Part model, mm, in its own coordinate system. A direction names the side the tool comes from. Give positions to 0.01 mm unless a question says otherwise; leave off trailing zeros. Write each loop counter-clockwise with the first axis right and the second up, starting at its lowest first coordinate (ties: lowest second). Pieces come first, ordered by that corner, then holes. Notation, with made-up numbers: M 34.25,14 L 85.25,14 A26 ccw 85.25,44 Z; hole C 87.5,4.5 d11. An arc over 180 degrees is marked long. Write item = value, one per line. Start each with the question number.
Autodesk Inventor part; units mm, degrees
ref_plane "YZ Plane" through (0, 0, 0) normal (1, 0, 0) x (0, 1, 0)
ref_plane "XZ Plane" through (0, 0, 0) normal (0, 1, 0) x (-1, 0, 0)
ref_plane "XY Plane" through (0, 0, 0) normal (0, 0, 1) x (1, 0, 0)
sketch "Sketch1" plane through (0, 0, 0) normal (0, 0, 1) x (1, 0, 0)
  line L0 (-20.5, -19.5) -> (20.5, -19.5)
  line L1 (20.5, -19.5) -> (20.5, 19.5)
  line L2 (20.5, 19.5) -> (-20.5, 19.5)
  line L3 (-20.5, 19.5) -> (-20.5, -19.5)
  line L4 (-20.5, -19.5) -> (20.5, 19.5) construction
  line L5 (20.5, -19.5) -> (-20.5, 19.5) construction
  line L6 (-17, -17) -> (17, -17) construction
  line L7 (17, -17) -> (17, 17) construction
  line L8 (17, 17) -> (-17, 17) construction
  line L9 (-17, 17) -> (-17, -17) construction
  line L10 (-17, -17) -> (17, 17) construction
  line L11 (17, -17) -> (-17, 17) construction
  circle A0 centre (-17, 17) radius 1.5
  circle A1 centre (17, 17) radius 1.5
  circle A2 centre (17, -17) radius 1.5
  circle A3 centre (-17, -17) radius 1.5
  point P0 (0, 0)
  dimension "d0" = 41
  dimension "d1" = 39
  dimension "d2" = 34
  dimension "d3" = 34
  dimension "d4" = 3
extrude "Extrusion1" add sketch "Sketch1" against normal blind 10
sketch "Sketch2" plane through (0, 0, 0) normal (0, 0, 1) x (1, 0, 0)
  line L0 (-14, -14) -> (14, -14)
  line L1 (14, -14) -> (14, 14)
  line L2 (14, 14) -> (-14, 14)
  line L3 (-14, 14) -> (-14, -14)
  line L4 (-14, -14) -> (14, 14) construction
  line L5 (14, -14) -> (-14, 14) construction
  point P0 (0, 0)
  dimension "d7" = 28
  dimension "d8" = 28
extrude "Extrusion2" add sketch "Sketch2" along normal blind 7
sketch "Sketch3" plane through (0, 0, 7) normal (0, 0, 1) x (1, 0, 0)
  circle A0 centre (0, 0) radius 7.1
  dimension "d11" = 14.2
extrude "Extrusion3" add sketch "Sketch3" along normal blind 20
sketch "Sketch4" plane through (0, 0, -10) normal (0, 0, -1) x (-1, 0, 0)
  line L0 (-20.5, 19.5) -> (-20.5, -19.5)
  line L1 (-20.5, 19.5) -> (-13.5, 19.5)
  line L2 (-13.5, 19.5) -> (-13.5, 12.5)
  line L3 (-13.5, 12.5) -> (-20.5, 12.5)
  line L4 (-20.5, 12.5) -> (-20.5, 19.5)
  line L5 (20.5, 19.5) -> (-20.5, 19.5)
  line L6 (20.5, 19.5) -> (13.5, 19.5)
  line L7 (13.5, 19.5) -> (13.5, 12.5)
  line L8 (13.5, 12.5) -> (20.5, 12.5)
  line L9 (20.5, 12.5) -> (20.5, 19.5)
  line L10 (20.5, 19.5) -> (20.5, -19.5)
  line L11 (20.5, -19.5) -> (13.5, -19.5)
  line L12 (13.5, -19.5) -> (13.5, -12.5)
  line L13 (13.5, -12.5) -> (20.5, -12.5)
  line L14 (20.5, -12.5) -> (20.5, -19.5)
  line L15 (-20.5, -19.5) -> (-13.5, -19.5)
  line L16 (-13.5, -19.5) -> (-13.5, -12.5)
  line L17 (-13.5, -12.5) -> (-20.5, -12.5)
  line L18 (-20.5, -12.5) -> (-20.5, -19.5)
  point P0 (0, 0)
  dimension "d14" = 7
extrude "Extrusion4" cut sketch "Sketch4" against normal blind 6.2
equation "\"d0\" = imx291ModuleWidth"
equation "\"d1\" = imx291ModuleLength"
equation "\"d2\" = imx291ModuleScrewWidthDistance"
equation "\"d3\" = imx291ModuleScrewLengthDistance"
equation "\"d4\" = screwDiameterHole"
equation "\"d5\" = imx291ModuleDepth"
equation "\"d7\" = lensBaseWidth"
equation "\"d8\" = lensBaseLength"
equation "\"d9\" = lensBaseDepth"
equation "\"d11\" = lensDiameter"
equation "\"d12\" = lensDepth"
equation "\"imx291ModuleWidth\" = 41"
equation "\"imx291ModuleLength\" = 39"
equation "\"imx291ModuleDepth\" = 10"
equation "\"imx291ModuleScrewWidthDistance\" = 34"
equation "\"imx291ModuleScrewLengthDistance\" = 34"
equation "\"screwDiameterHole\" = 3"
equation "\"lensBaseWidth\" = 28"
equation "\"lensBaseLength\" = 28"
equation "\"lensBaseDepth\" = 7"
equation "\"lensDiameter\" = 14.2"
equation "\"lensDepth\" = 20"
properties part number "imx291CameraModule"
Q1. Drop flat-ended pins along their axis: P1, Ø3.5, axis at x = -17, y = -17, coming from the +Z side; P2, Ø11.5, axis at x = 10, y = -8.5, coming from the +Z side; P3, Ø7, axis at y = 16, z = -6, coming from the -X side; P4, Ø1.5, axis at y = 9, z = 1, coming from the -X side. Give the stop position or say it passes through.
Q2. Probe line 1 along Y through (x, z) = (-17, -2.3); line 2 along Z through (x, y) = (15.5, 2); line 3 along Z through (x, y) = (-12, 6.5). List the from-to ranges inside material, lowest first.
Q3. Tool access for faces 1 (the face through (-13.5, -16, -7)), 2 (the face through (-13.5, 16, -7)), 3 (the face through (-0.92, -7.04, 16.86)): list every direction of +Z, -Z, +X, -X, +Y, -Y with a clear straight run to the whole face (end or side of a thin tool).
Q4. Two-plate mould, pull along X, no slides. Class faces 4 (the face through (0, 14, 3)), 5 (the face through (-14, 0, 3)), 6 (the face through (-18.5, -16.93, -1.87)): +X half, -X half, draft (parallel to the pull), parting line (faces both ways), or undercut.
Q5. Slice it at D-D (y = -9.5). Give the cut face in (x, z).
Q6. Slice it at B-B (y = 17). Give the cut face in (x, z), and give its area (3 significant figures).
Q7. Slice it at C-C (x = 0). Give the cut face in (y, z), and give its area (3 significant figures).
Q8. Slice it at A-A (x = 17). Give the cut face in (y, z).
Working result:
q1.P1 = 0
q1.P2 = 7
q1.P3 = -20.5
q1.P4 = -14
q2.line_1 = -19.5 to -18.5, -15.5 to 15.5, 18.5 to 19.5
q2.line_2 = -10 to 0
q2.line_3 = -10 to 7
q3.face_1 = -Z, -X, -Y
q3.face_2 = -Z, -X, +Y
q3.face_3 = +Z
q4.face_4 = draft
q4.face_5 = -X half
q4.face_6 = undercut
q5.outline = M -20.5,-10 L 20.5,-10 L 20.5,0 L 14,0 L 14,7 L -14,7 L -14,0 L -20.5,0 Z
q6.outline = M -20.5,-3.8 L -18.5,-3.8 L -18.5,0 L -20.5,0 Z; M -15.5,-3.8 L -13.5,-3.8 L -13.5,-10 L 13.5,-10 L 13.5,-3.8 L 15.5,-3.8 L 15.5,0 L -15.5,0 Z; M 18.5,-3.8 L 20.5,-3.8 L 20.5,0 L 18.5,0 Z
q6.area = 300 mm2
q7.outline = M -19.5,-10 L 19.5,-10 L 19.5,0 L 14,0 L 14,7 L 7.1,7 L 7.1,27 L -7.1,27 L -7.1,7 L -14,7 L -14,0 L -19.5,0 Z
q7.area = 870 mm2
q8.outline = M -19.5,-3.8 L -18.5,-3.8 L -18.5,0 L -19.5,0 Z; M -15.5,-3.8 L -12.5,-3.8 L -12.5,-10 L 12.5,-10 L 12.5,-3.8 L 15.5,-3.8 L 15.5,0 L -15.5,0 Z; M 18.5,-3.8 L 19.5,-3.8 L 19.5,0 L 18.5,0 Z
